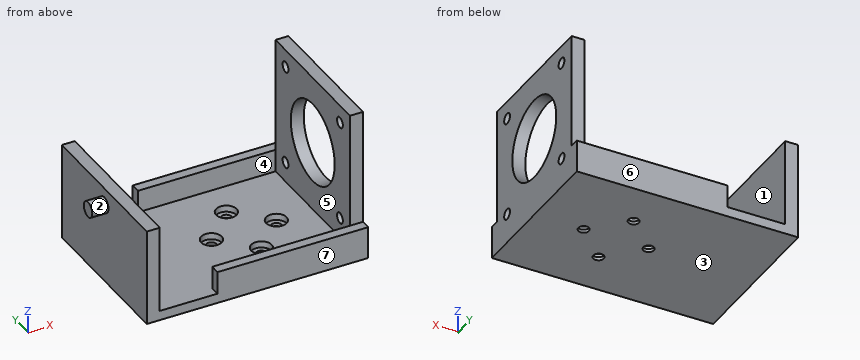
from build123d import *

# Parameters (mm, degrees)
SKETCH_1_W          = 42.4
SKETCH_1_H          = 42.4
SKETCH_1_R          = 3.15
EXTRUDE_1_DEPTH     = 3
SKETCH_1_3_R        = 3.15
SKETCH_1_3_R_2      = 1.65
EXTRUDE_2_DEPTH     = 1
SKETCH_2_W          = 4
SKETCH_2_H          = 42.4
EXTRUDE_3_DEPTH     = 45.7
SKETCH_3_R          = 1.65
SKETCH_3_R_2        = 12.5
CUT_EXTRUDE_2_DEPTH = 45.2
SKETCH_4_W          = 46.4
SKETCH_4_H          = 3
EXTRUDE_4_DEPTH     = 10
SKETCH_9_W          = 17.8
SKETCH_9_H          = 48.4
EXTRUDE_8_DEPTH     = 3
SKETCH_10_W         = 4
SKETCH_10_H         = 48.4
EXTRUDE_9_DEPTH     = 30
EXTRUDE_START       = -43
SKETCH_11_R         = 2.4
EXTRUDE_10_DEPTH    = 5


with BuildPart() as part:
    # 草图1 → 凸台-拉伸1 (new body)
    with BuildSketch(Plane.XY):
        Rectangle(SKETCH_1_W, SKETCH_1_H)
        with Locations((-10, 0)):
            Circle(SKETCH_1_R, mode=Mode.SUBTRACT)
        with Locations((0, -10)):
            Circle(SKETCH_1_R, mode=Mode.SUBTRACT)
        with Locations((10, 0)):
            Circle(SKETCH_1_R, mode=Mode.SUBTRACT)
        with Locations((0, 10)):
            Circle(SKETCH_1_R, mode=Mode.SUBTRACT)
    extrude(amount=EXTRUDE_1_DEPTH)

    # 草图1<3> → 凸台-拉伸2 (add)
    # profile 1 of 4: a face of its own
    with BuildSketch(Plane.XY):
        with Locations((-10, 0)):
            Circle(SKETCH_1_3_R)
        with Locations((-10, 0)):
            Circle(SKETCH_1_3_R_2, mode=Mode.SUBTRACT)
    # profile 2 of 4: a face of its own
    with BuildSketch(Plane.XY):
        with Locations((0, 10)):
            Circle(SKETCH_1_3_R)
        with Locations((0, 10)):
            Circle(SKETCH_1_3_R_2, mode=Mode.SUBTRACT)
    # profile 3 of 4: a face of its own
    with BuildSketch(Plane.XY):
        with Locations((10, 0)):
            Circle(SKETCH_1_3_R)
        with Locations((10, 0)):
            Circle(SKETCH_1_3_R_2, mode=Mode.SUBTRACT)
    # profile 4 of 4: a face of its own
    with BuildSketch(Plane.XY):
        with Locations((0, -10)):
            Circle(SKETCH_1_3_R)
        with Locations((0, -10)):
            Circle(SKETCH_1_3_R_2, mode=Mode.SUBTRACT)
    extrude(amount=EXTRUDE_2_DEPTH)

    # 草图2 → 凸台-拉伸3 (add)
    with BuildSketch(Plane.XY):
        with Locations((23.2, 0)):
            Rectangle(SKETCH_2_W, SKETCH_2_H)
    extrude(amount=EXTRUDE_3_DEPTH)

    # 草图3 → 切除-拉伸2 (cut)
    with BuildSketch(Plane(origin=(0, 0, 0), x_dir=(0, 0, -1), z_dir=(1, 0, 0))):
        with Locations(Location((-9.2, -15.5, 0), (0, 0, 180))):
            Circle(SKETCH_3_R)
        with Locations(Location((-40.2, -15.5, 0), (0, 0, 180))):
            Circle(SKETCH_3_R)
        with Locations(Location((-40.2, 15.5, 0), (0, 0, 180))):
            Circle(SKETCH_3_R)
        with Locations(Location((-9.2, 15.5, 0), (0, 0, 180))):
            Circle(SKETCH_3_R)
        with Locations(Location((-24.7, 0, 0), (0, 0, 180))):
            Circle(SKETCH_3_R_2)
    extrude(amount=CUT_EXTRUDE_2_DEPTH, mode=Mode.SUBTRACT)

    # 草图4 → 凸台-拉伸4 (add)
    with BuildSketch(Plane.XY):
        with Locations((2, -22.7)):
            Rectangle(SKETCH_4_W, SKETCH_4_H)
        with Locations((2, 22.7)):
            Rectangle(SKETCH_4_W, SKETCH_4_H)
    extrude(amount=EXTRUDE_4_DEPTH)

    # 草图9 → 凸台-拉伸8 (add)
    with BuildSketch(Plane.XY):
        with Locations((-30.1, 0)):
            Rectangle(SKETCH_9_W, SKETCH_9_H)
    extrude(amount=EXTRUDE_8_DEPTH)

    # 草图10 → 凸台-拉伸9 (add)
    with BuildSketch(Plane.XY):
        with Locations((-41, 0)):
            Rectangle(SKETCH_10_W, SKETCH_10_H)
    extrude(amount=EXTRUDE_9_DEPTH)

    # 草图11 → 凸台-拉伸10 (add)
    with BuildSketch(Plane(origin=(0, 0, 0), x_dir=(0, 0, -1), z_dir=(1, 0, 0)).offset(EXTRUDE_START)):
        with Locations((-24.7, 0)):
            Circle(SKETCH_11_R)
    extrude(amount=-EXTRUDE_10_DEPTH)


solid = part.part
CAD build for the part. Positions are in the model's coordinates, mm. Face numbers are marked on the shaded views. A direction names the side the tool comes from. Give positions to 0.01 mm unless a question says otherwise; leave off trailing zeros. Write each loop counter-clockwise with the first axis right and the second up, starting at its lowest first coordinate (ties: lowest second). Pieces come first, ordered by that corner, then holes. Notation, with made-up numbers: (41.25, 0) - (93.25, 0) arc R23 cw to (93.25, 32) - close; hole circle Ø11 at (52.25, 42.25). An arc over 180 degrees is marked (long way). Put each result on its own line as item: value.
(1) Saw through at C-C (z = 9.2). List the corners of the cut face in (x, y), then the cut area to 3 significant figures.
Working result:
outline: (-43, -24.2) - (-39, -24.2) - (-39, 24.2) - (-43, 24.2) - close; (-21.2, -24.2) - (25.2, -24.2) - (25.2, -17.15) - (21.2, -17.15) - (21.2, -21.2) - (-21.2, -21.2) - close; (-21.2, 21.2) - (21.2, 21.2) - (21.2, 17.15) - (25.2, 17.15) - (25.2, 24.2) - (-21.2, 24.2) - close; (21.2, -13.85) - (25.2, -13.85) - (25.2, 13.85) - (21.2, 13.85) - close
area: 615 mm^2
(2) Saw through at B-B (y = 0). Count the separate pieces of the cut face and the enclosed holes in it, then the cut area to 3 significant figures.
Working result:
separate pieces: 4
enclosed holes: 0
area: 376 mm^2
(3) Saw through at D-D (y = 10). List the corners of the cut face in (x, z).
Working result:
outline: (-43, 0) - (-1.65, 0) - (-1.65, 1) - (-3.15, 1) - (-3.15, 3) - (-39, 3) - (-39, 30) - (-43, 30) - close; (1.65, 0) - (25.2, 0) - (25.2, 17.2) - (21.2, 17.2) - (21.2, 3) - (3.15, 3) - (3.15, 1) - (1.65, 1) - close; (21.2, 32.2) - (25.2, 32.2) - (25.2, 45.7) - (21.2, 45.7) - close
(4) Drop flat-ended pins along their axis: pin 1 Ø5.5 at (y, z) = (15.5, 40.2) entering from -X; pin 2 Ø7 at (x, y) = (-9, -0.5) entering from +Z; pin 3 Ø5.5 at (x, y) = (0, -10) entering from +Z. Give the stop position or say it passes through.
Working result:
pin 1: x = 21.2
pin 2: z = 3
pin 3: z = 1
(5) Tool access for the marked faces 1, 2, 3 and 4: list every direction of +Z, -Z, +X, -X, +Y, -Y with a clear straight run to the whole face (end or side of a thin tool).
Working result:
face 1: +Z, +Y, -Y
face 2: -X
face 3: -Z, +X, -X, +Y, -Y
face 4: +Z
(6) Wall check: L1, parallel to Y at x = 22.65, z = 40.2; L2, parallel to Y at x = 22.3, z = 9.2; L3, parallel to X at y = 16, z = 29.5. Give the ranges that are in metal, low to high.
Working result:
L1: -21.2 to -17.15, -13.85 to 13.85, 17.15 to 21.2
L2: -24.2 to -17.15, -13.85 to 13.85, 17.15 to 24.2
L3: -43 to -39, 21.2 to 25.2
(7) Pull direction Y, two halves, no side cores. Call the marked faces 5, 6 and 7: released by +Y, released by -Y, zero draft, split by the parting line, or undercut.
Working result:
face 5: undercut
face 6: released by +Y
face 7: released by -Y
(8) Saw through at A-A (x = 10). List the corners of the cut face in (y, z), then the cut area to 3 significant figures.
Working result:
outline: (-24.2, 0) - (-1.65, 0) - (-1.65, 1) - (-3.15, 1) - (-3.15, 3) - (-21.2, 3) - (-21.2, 10) - (-24.2, 10) - close; (1.65, 0) - (24.2, 0) - (24.2, 10) - (21.2, 10) - (21.2, 3) - (3.15, 3) - (3.15, 1) - (1.65, 1) - close
area: 171 mm^2
